Source: three-view drawing plus pictorial views. Frame: mm from the lowest corner of the part. A direction names the side the tool comes from. Give positions to 0.01 mm unless a question says otherwise; leave off trailing zeros. Order: outer loops, then holes, each group sorted by start corner. A loop starts at its lowest first (then second) coordinate and runs counter-clockwise, first axis right, second up.
1) First-contact query: P1, Ø21, axis at x = 39.5, z = 48.5, coming from the +Y side; P2, Ø12, axis at y = 101.5, z = 41.5, coming from the -X side; P3, Ø8, axis at x = 62, z = 27, coming from the +Y side. Flat tips, straight axial feed; report the tip coordinate or a pass-through.
2) Material intervals for line 1 (X direction, y = 27, z = 8.5); line 2 (Z direction, x = 61, y = 39); line 3 (X direction, y = 20.5, z = 4), sorted ascending.
3) Draft query along Y for the marked faces 1, 2 and 3. Return one class per face: released by +Y, released by -Y, zero draft, split by the parting line, or undercut.
4) Section B-B, the plane y = 75. Give the number of separate pieces and of enclosed holes in the cut face, plus the area to 3 significant figures.
5) Section A-A, the plane z = 46.5. Return loops of the section in (x, y).
6) Section C-C, the plane x = 18.5. Return loops of the section in (y, z).
7) Section D-D, the plane z = 5. Return loops of the section in (x, y), plus the area to 4 significant figures.
8) Access query for the marked faces 4 and 5. Directions: +Z, -Z, +X, -X, +Y, -Y. A direction counts if a zero-diameter tool reaches every point of the face in a straight line with its end or side. Return the directions, or none.
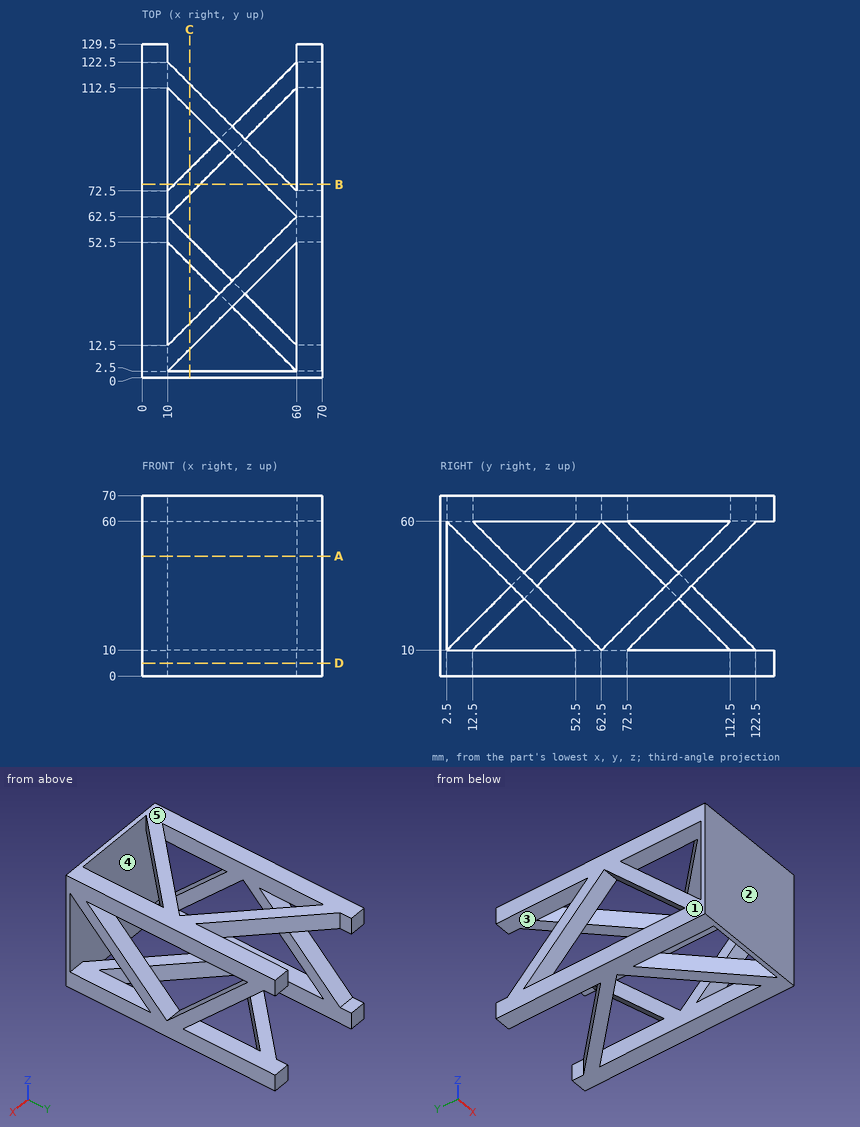
From the geometry:
1. P1: stops at y = 2.5
1. P2: stops at x = 60
1. P3: stops at y = 93.5
2. line 1: x = 0 to 10, 35.5 to 45.5, 60 to 70
2. line 2: z = 0 to 10, 23.5 to 33.5, 60 to 70
2. line 3: x = 0 to 10, 42 to 52, 60 to 70
3. face 1: zero draft
3. face 2: released by -Y
3. face 3: undercut
4. separate pieces: 8
4. enclosed holes: 0
4. area: 800 mm2
5. outline: (0, 0) - (70, 0) - (70, 2.5) - (0, 2.5) - close; (0, 39) - (10, 39) - (10, 49) - (0, 49) - close; (0, 76) - (10, 76) - (10, 86) - (0, 86) - close; (60, 16) - (70, 16) - (70, 26) - (60, 26) - close; (60, 99) - (70, 99) - (70, 109) - (60, 109) - close
6. outline: (0, 0) - (2.5, 0) - (2.5, 70) - (0, 70) - close; (11, 60) - (21, 60) - (21, 70) - (11, 70) - close; (44, 0) - (54, 0) - (54, 10) - (44, 10) - close; (71, 0) - (81, 0) - (81, 10) - (71, 10) - close; (104, 60) - (114, 60) - (114, 70) - (104, 70) - close
7. outline: (0, 0) - (70, 0) - (70, 129.5) - (60, 129.5) - (60, 122.5) - (10, 72.5) - (10, 129.5) - (0, 129.5) - close; hole (10, 2.5) - (60, 2.5) - (10, 52.5) - close; hole (10, 62.5) - (60, 12.5) - (60, 112.5) - close
7. area: 3,715 mm2
8. face 4: none
8. face 5: +Z, +X, -X, +Y, -Y
